The listing builds one solid part. Answer for the finished solid, in the listing's coordinates (mm). A direction names the side the tool comes from. Give positions to 0.01 mm unless a question says otherwise; leave off trailing zeros. Write each loop counter-clockwise with the first axis right and the second up, starting at its lowest first coordinate (ties: lowest second). Pieces come first, ordered by that corner, then holes.
Autodesk Inventor part; units mm, degrees
ref_plane "YZ Plane" through (0, 0, 0) normal (1, 0, 0) x (0, 1, 0)
ref_plane "XZ Plane" through (0, 0, 0) normal (0, 1, 0) x (-1, 0, 0)
ref_plane "XY Plane" through (0, 0, 0) normal (0, 0, 1) x (1, 0, 0)
sketch "Sketch1" plane through (0, 0, 0) normal (0, 0, 1) x (1, 0, 0)
  circle A0 centre (0, 0) radius 10
  dimension "d0" = 20
extrude "Extrusion1" add sketch "Sketch1" along normal blind 10
sketch "Sketch2" plane through (0, 0, 10) normal (0, 0, 1) x (1, 0, 0)
  point P0 (0, 0)
  point P1 (0, 0)
hole "Hole1" at (0, 0, 10) direction (0, 0, -1) diameter 5 end through all
chamfer "Chamfer1" distance 0.5 angle 45 1 edges at (0, 2.5, 10)
sketch "Sketch3" plane through (0, 0, 10) normal (0, 0, 1) x (1, 0, 0)
  circle A0 centre (0, 0) radius 10
  line L0 (-10, 0) -> (-9, 0)
  line L1 (-9, 0) -> (-9, 4.3589)
  line L2 (-9, 4.3589) -> (-10, 4.3589)
  line L3 (-10, 4.3589) -> (-10, 0)
  line L4 (-10, 0) -> (-9, 0)
  line L5 (-9, 0) -> (-9, -4.4002)
  line L6 (-9, -4.4002) -> (-10, -4.4002)
  line L7 (-10, -4.4002) -> (-10, 0)
  line L8 (10.026, 0) -> (9.026, 0)
  line L9 (9.026, 0) -> (9.026, 4.3589)
  line L10 (9.026, 4.3589) -> (10.026, 4.3589)
  line L11 (10.026, 4.3589) -> (10.026, 0)
  line L12 (10.026, 0) -> (9.026, 0)
  line L13 (9.026, 0) -> (9.026, -4.4002)
  line L14 (9.026, -4.4002) -> (10.026, -4.4002)
  line L15 (10.026, -4.4002) -> (10.026, 0)
  dimension "d13" = 1
  dimension "d14" = 1
  dimension "d15" = 1
extrude "Extrusion2" cut sketch "Sketch3" against normal blind 10 contours L1 L0 A0 | L0 L5 A0 | A0 L5 L6 L7 | L9 L10 L11 L8 A0 | A0 L8 L9 | L8 L15 L14 L13 A0 | A0 L13 L8
sketch "Sketch4" plane through (9.026, -4.3048, 10) normal (1, 0, 0) x (0, 0, -1)
  line L0 (10, 4.3048) -> (5, 4.3048)
  line L1 (0.5, 1.8048) -> (0.5, 6.8048)
  dimension "d18" = 5
hole "Hole2" at (9.026, 0, 5) direction (-1, 0, 0) diameter 3 end through all
sketch "Sketch5" plane through (9.026, -4.3048, 10) normal (1, 0, 0) x (0, 0, -1)
  circle A0 centre (5, 4.3048) radius 1.5
  point P0 (10, 4.3048)
hole "Hole3" at (9.026, 0, 5) direction (-1, 0, 0) diameter 3.5 depth 3.5
sketch "Sketch6" plane through (-9, -4.3589, 10) normal (-1, 0, 0) x (0, 0, 1)
  circle A0 centre (-5, 4.3589) radius 1.5
  point P0 (-10, 4.3589)
hole "Hole4" at (-9, 0, 5) direction (1, 0, 0) diameter 3.5 depth 3.5
sketch "Sketch7" plane through (0, 0, 0) normal (0, 0, -1) x (-1, 0, 0)
  line L0 (0, 0) -> (-9.026, 0)
  line L1 (-9.026, 0) -> (-9.026, 18)
  line L2 (-9.026, 18) -> (0, 18)
  line L3 (0, 18) -> (0, 0)
  line L4 (0, 0) -> (-9.026, 0)
  line L5 (-9.026, 0) -> (-9.026, -18)
  line L6 (-9.026, -18) -> (0, -18)
  line L7 (0, -18) -> (0, 0)
  line L8 (0, 18) -> (23, 18)
  line L9 (23, 18) -> (23, -18)
  line L10 (23, -18) -> (0, -18)
  line L11 (0, -18) -> (0, 18)
  dimension "d40" = 9.026
  dimension "d41" = 18
  dimension "d42" = 18
  dimension "d43" = 23
extrude "Extrusion3" add sketch "Sketch7" along normal blind 3
sketch "Sketch8" plane through (0, 0, -3) normal (0, 0, -1) x (-1, 0, 0)
  line L0 (23, 18) -> (-9.026, 18)
  line L1 (-9.026, -18) -> (23, -18)
  line L2 (23, 18) -> (20, 18)
  line L3 (20, 18) -> (20, -18)
  line L4 (20, -18) -> (23, -18)
  line L5 (23, -18) -> (23, 18)
  point P0 (0, 0)
  dimension "d46" = 3
extrude "Extrusion4" add sketch "Sketch8" along normal blind 50
sketch "Sketch9" plane through (-20, -18, -3) normal (1, 0, 0) x (0, 0, -1)
  line L0 (0, 0) -> (0, 36)
  line L1 (0, 36) -> (25, 36)
  line L2 (-3, 36) -> (50, 36)
  line L3 (25, 36) -> (25, 18)
  line L4 (-3, 0) -> (50, 0)
  line L5 (25, 18) -> (39.5, 18)
  line L6 (39.5, 18) -> (39.5, 31.9)
  line L7 (39.5, 31.9) -> (25, 31.9)
  line L8 (25, 31.9) -> (25, 18)
  line L9 (25, 18) -> (39.5, 18)
  line L10 (39.5, 18) -> (39.5, 4.1)
  line L11 (39.5, 4.1) -> (25, 4.1)
  line L12 (25, 4.1) -> (25, 18)
  line L13 (25, 18) -> (10.5, 18)
  line L14 (10.5, 18) -> (10.5, 31.9)
  line L15 (10.5, 31.9) -> (25, 31.9)
  line L16 (25, 31.9) -> (25, 18)
  line L17 (25, 18) -> (10.5, 18)
  line L18 (10.5, 18) -> (10.5, 4.1)
  line L19 (10.5, 4.1) -> (25, 4.1)
  line L20 (25, 4.1) -> (25, 18)
  point P0 (-3, 18)
  dimension "d49" = 25
  dimension "d50" = 18
  dimension "d51" = 14.5
  dimension "d52" = 13.9
  dimension "d53" = 13.9
  dimension "d54" = 14.5
hole "Hole5" at (-20, 13.9, -13.5) at (-20, 13.9, -42.5) at (-20, -13.9, -42.5) at (-20, -13.9, -13.5) direction (-1, 0, 0) diameter 3.5 end through all
sketch "Sketch10" plane through (0, 0, -3) normal (0, 0, -1) x (-1, 0, 0)
  line L0 (-9.026, -18) -> (23, -18)
  circle A0 centre (0, 0) radius 29.2062
  circle A1 centre (0, 0) radius 2.5
  circle A2 centre (0, 0) radius 31.206
  dimension "d62" = 62.412
extrude "Extrusion5" add sketch "Sketch10" against normal blind 3.175 contours A0 | A2
sketch "Sketch11" plane through (0, 0, -3) normal (0, 0, -1) x (-1, 0, 0)
  line L0 (23, -18) -> (23, 18)
  circle A0 centre (0, 0) radius 29.2062
  line L1 (23, 18) -> (-23, 18)
  line L2 (-23, 18) -> (-23, -18)
  line L3 (-23, -18) -> (23, -18)
  line L4 (23, -18) -> (23, 18)
  circle A1 centre (0, 0) radius 2.5
  line L5 (0, 0) -> (0, 23)
  line L6 (0, 23) -> (11.5, 23)
  line L7 (11.5, 23) -> (-11.5, 23)
  line L8 (-11.5, 23) -> (-11.5, -23)
  line L9 (-11.5, -23) -> (11.5, -23)
  line L10 (11.5, -23) -> (11.5, 23)
  dimension "d65" = 23
  dimension "d66" = 11.5
  dimension "d67" = 23
  dimension "d68" = 46
hole "Hole6" at (11.5, 23, -3) at (-11.5, 23, -3) at (11.5, -23, -3) at (-11.5, -23, -3) direction (0, 0, 1) diameter 3 depth 3.5
sketch "Sketch12" plane through (-20, -18, -3) normal (1, 0, 0) x (0, 0, -1)
  line L0 (0, 0) -> (0, 36)
  line L1 (50, 0) -> (50, 36)
  point P0 (-3, 18)
  point P1 (25, 18)
sketch "Sketch13" plane through (0, 0, 0.175) normal (0, 0, 1) x (1, 0, 0)
  arc A0 (9.026, 4.3048) -> (-9, 4.3589) centre (0, 0) ccw
  line L0 (0, 10) -> (6, 10)
  line L1 (6, 10) -> (6, 14)
  line L2 (6, 14) -> (0, 14)
  line L3 (0, 14) -> (0, 10)
  line L4 (6, 14) -> (-6, 14)
  line L5 (-6, 14) -> (-6, 10)
  line L6 (-6, 10) -> (6, 10)
  line L7 (6, 10) -> (6, 14)
  dimension "d76" = 6
  dimension "d77" = 4
  dimension "d78" = 12
extrude "Extrusion6" cut sketch "Sketch13" against normal blind 3.175
fillet "Fillet1" radius 2 4 edges at (-6, 14, -1.4125) (6, 14, -1.4125) (6, 10, -1.4125) (-6, 10, -1.4125)
sketch "Sketch14" plane through (-23, -18, -3) normal (-1, 0, 0) x (0, 0, 1)
  circle A0 centre (-39.5, 31.9) radius 1.75
  circle A1 centre (-10.5, 4.1) radius 1.75
  line L0 (-39.5, 31.9) -> (-10.5, 4.1)
  circle A2 centre (-39.5, 4.1) radius 1.75
  line L1 (-10.5, 4.1) -> (-39.5, 4.1)
  circle A3 centre (-10.5, 31.9) radius 1.75
  line L2 (-39.5, 4.1) -> (-10.5, 31.9)
  point P0 (3, 18)
  point P1 (-25, 18)
hole "Hole7" at (-23, 0, -28) direction (1, 0, 0) diameter 5 end through all
properties part number "LidarLiteV3Mount"
Item 1: A cutting plane is placed at B-B, the plane y = -23. Give the vertices of the cut face in (x, z) (3 decimals).
Conclusion:
outline: (-21.091, -3) - (-13, -3) - (-13, 0.175) - (-21.091, 0.175) - close; (-10, -3) - (10, -3) - (10, 0.175) - (-10, 0.175) - close; (13, -3) - (21.091, -3) - (21.091, 0.175) - (13, 0.175) - close
Item 2: A cutting plane is placed at D-D, the plane z = 1.5. Give the vertices of the cut face in (x, y), plus the area to 3 significant figures.
Conclusion:
outline: (-9, -4.36) arc R10 ccw to (9.03, -4.3) - (9.03, 4.3) arc R10 ccw to (-9, 4.36) - close; hole circle Ø5 at (0, 0)
area: 283 mm2
Item 3: Which of the six approach directions +Z, -Z, +X, -X, +Y, -Y give full straight-line access (tool end or side, diameter ignored) to faces 1 (the face through (0, 10, -1)), 2 (the face through (0, 0, 0)), 3 (the face through (0, 10, 5)), 4 (the face through (-23, -4, -28)), 5 (the face through (9.026, -2, 5))?
Conclusion:
face 1: +Z, -Z
face 2: +Z
face 3: +Z, +Y
face 4: -Z, -X, +Y, -Y
face 5: +Z, +X, +Y, -Y
Item 4: A cutting plane is placed at C-C, the plane x = -11.5. Give the vertices of the cut face in (y, z) (3 decimals).
Conclusion:
outline: (-29.01, -3) - (-24.5, -3) - (-24.5, 0.175) - (-29.01, 0.175) - close; (-21.5, -3) - (21.5, -3) - (21.5, 0.175) - (-21.5, 0.175) - close; (24.5, -3) - (29.01, -3) - (29.01, 0.175) - (24.5, 0.175) - close
Item 5: Each of these flat-tipped pins is pushed along its axis until it touches: P1, Ø3, axis at y = 13.9, z = -13.5, coming from the +X side; P2, Ø4, axis at x = -18.5, z = -31, coming from the +Y side; P3, Ø6, axis at y = 15.5, z = -29, coming from the -X side; P4, Ø6, axis at x = 0, y = 0, coming from the -Z side. Where does it stop, or does it pass through?
Conclusion:
P1: passes through
P2: stops at y = 18
P3: stops at x = -23
P4: stops at z = -3
Item 6: Consider probe 1 along Z at (x, y) = (-22.2, -13.9) (3 decimals); probe 2 along Y at (x, z) = (-11.5, -0.65); probe 3 along X at (y, z) = (-23, -2.3). Determine where each line is inside the solid, lowest interval first.
Conclusion:
probe 1: z = -53 to -44.25, -40.75 to -15.25, -11.75 to 0.175
probe 2: y = -29.01 to -24.5, -21.5 to 21.5, 24.5 to 29.01
probe 3: x = -21.09 to -13, -10 to 10, 13 to 21.09
Item 7: Determine the mould class of faces 6 (the face through (-2.1, 2.4, 10)), 7 (the face through (-21, -18, -28)), 8 (the face through (5.43, 10.6, -1.43)) for opening direction Y: pulls with the +Y half, pulls with the -Y half, needs draft (parallel to the pull), parting line crosses it, or undercut.
Conclusion:
face 6: needs draft
face 7: pulls with the -Y half
face 8: undercut
Item 8: A cutting plane is placed at A-A, the plane z = -29.5. Give the vertices of the cut face in (x, y).
Conclusion:
outline: (-23, -18) - (-20, -18) - (-20, -2) - (-23, -2) - close; (-23, 2) - (-20, 2) - (-20, 18) - (-23, 18) - close
